Source: CAD feature listing. Evaluate the final solid. Frame: model axes, mm. A direction names the side the tool comes from. Give positions to 0.01 mm unless a question says otherwise; leave off trailing zeros. Loops run counter-clockwise (first coordinate to the right, second up) from the corner with the lowest first, then second, coordinate; pieces in that order, holes last. Notation, with made-up numbers: M 52,-9 L 68,-9 A18 cw 68,21 Z; hole C -20,57 d11. An arc over 180 degrees is marked long. Put each result on its own line as item: value. Start each with the question number.
```python
from build123d import *

# Parameters (mm, degrees)
POSICIONAMENTOS_R               = 6.8994
BASE_DEPTH                      = 3
BASE_DENTE_DEPTH                = 3
RAIO_DENTE_R                    = 0.778916794
PADR_OCIRCULAR1_COUNT           = 10
RAIO_DENTE_OF_PADR_OCIRCULAR1_R = 0.778916794
RESSALTO_EXTRUS_O3_DEPTH        = 3
FURO_DE_DI_METRO_3_0_3_1_D      = 3
FILETE2_R                       = 5
FILETE3_R                       = 13
FILETE4_R                       = 1


with BuildPart() as part:
    # Posicionamentos → Base (new body)
    with BuildSketch(Plane.XY):
        Circle(POSICIONAMENTOS_R)
    extrude(amount=BASE_DEPTH)

    # Dente → Base Dente (add, through all)
    with BuildSketch(Plane.XY):
        with BuildLine():
            Line((1.480256779, 8.326682401), (1.207591527, 6.792896515))
            ThreePointArc((1.207591527, 6.792896515), (0, 6.8994), (-1.207591527, 6.792896515))
            Line((-1.207591527, 6.792896515), (-1.480256779, 8.326682401))
            ThreePointArc((-1.480256779, 8.326682401), (-1.476621376, 8.612123538), (-1.407910185, 8.889195065))
            ThreePointArc((-1.407910185, 8.889195065), (-1.05050148, 9.903958065), (-0.441648539, 10.79096597))
            ThreePointArc((-0.441648539, 10.79096597), (0, 10.8), (0.441648539, 10.79096597))
            ThreePointArc((0.441648539, 10.79096597), (1.05050148, 9.903958065), (1.407910185, 8.889195065))
            ThreePointArc((1.407910185, 8.889195065), (1.476621376, 8.612123538), (1.480256779, 8.326682401))
        make_face()
    base_dente = extrude(amount=BASE_DENTE_DEPTH)

    # Raio Dente
    raio_dente_edges = [part.edges().sort_by_distance(p)[0] for p in [
        (-1.207591527, 6.792896515, 1.5),
        (1.207591527, 6.792896515, 1.5),
    ]]
    fillet(raio_dente_edges, radius=RAIO_DENTE_R)

    # PadrãoCircular1: Base Dente ×10 about axis, 2 skipped
    padr_ocircular1_axis = Axis((0, 0, 0), (0, 0, -1))
    add([base_dente.rotate(padr_ocircular1_axis, i * 360 / PADR_OCIRCULAR1_COUNT) for i in range(1, PADR_OCIRCULAR1_COUNT) if i not in (7, 8)])

    # Raio Dente of PadrãoCircular1
    raio_dente_of_padr_ocircular1_edges = [part.edges().sort_by_distance(p)[0] for p in [
        (3.015802325, 6.205373212, 1.5),
        (4.969726459, 4.785764232, 1.5),
        (6.087262191, 3.247608255, 1.5),
        (6.833594799, 0.950632674, 1.5),
        (6.833594799, -0.950632674, 1.5),
        (6.087262191, -3.247608255, 1.5),
        (4.969726459, -4.785764232, 1.5),
        (3.015802325, -6.205373212, 1.5),
        (1.207591527, -6.792896515, 1.5),
        (-1.207591527, -6.792896515, 1.5),
        (-3.015802325, -6.205373212, 1.5),
        (-4.969726459, -4.785764232, 1.5),
        (-4.969726459, 4.785764232, 1.5),
        (-3.015802325, 6.205373212, 1.5),
    ]]
    fillet(raio_dente_of_padr_ocircular1_edges, radius=RAIO_DENTE_OF_PADR_OCIRCULAR1_R)

    # Braço → Ressalto-extrusão3 (add, through all)
    with BuildSketch(Plane.XY):
        Polygon((0, 4), (-25, 4), (-38, -9), (-25.102702489, -7.416410988), (-21.686291501, -4), (0, -4), align=None)
    extrude(amount=RESSALTO_EXTRUS_O3_DEPTH)

    # Furo de diâmetro Ø3.0 (3)1 (through all)
    with Locations(Plane.XY.offset(3)):
        with Locations((0, 0)):
            Hole(FURO_DE_DI_METRO_3_0_3_1_D / 2)

    # Filete2
    filete2_edges = [part.edges().sort_by_distance(p)[0] for p in [
        (-21.686291501, -4, 1.5),
    ]]
    fillet(filete2_edges, radius=FILETE2_R)

    # Filete3
    filete3_edges = [part.edges().sort_by_distance(p)[0] for p in [
        (-25, 4, 1.5),
    ]]
    fillet(filete3_edges, radius=FILETE3_R)

    # Filete4
    filete4_edges = [part.edges().sort_by_distance(p)[0] for p in [
        (-25.102702489, -7.416410988, 1.5),
        (-38, -9, 1.5),
    ]]
    fillet(filete4_edges, radius=FILETE4_R)


solid = part.part
```
1. Section C-C, the plane y = 2.5. Output: boundary loops of the cut face in (x, z), plus the area to 3 significant figures.
2. Ray query, line 1 (Y direction, x = 0, z = 1.5); line 2 (X direction, y = 4.75, z = 2.2); line 3 (X direction, y = 8.75, z = 1.25). Return the intervals inside material, ascending.
3. Section B-B, the plane x = -17. Output: boundary loops of the cut face in (y, z).
4. Pull-direction query (X, two-part tool) for faces 5 (the face through (-24.66, 2.98, 1.52)), 6 (the face through (-30.35, -8.06, 1.48)), 7 (the face through (10.27, 3.34, 1.48)); classes: released by +X, released by -X, zero draft, split by the parting line, or undercut.
5. Section A-A, the plane x = 0. Output: boundary loops of the cut face in (y, z).
6. Set-up query: faces 1 (the face through (4.985, -8.637, 1.479)), 2 (the face through (-32, -3, 1)), 3 (the face through (1.408, -7.918, 1.479)), 4 (the face through (4.958, 8.623, 1.479)). Return all of +Z, -Z, +X, -X, +Y, -Y with unobstructed straight access to the full face (end or side cutting, diameter ignored); none if empty.
7. Contact query for flat-ended pins moving along their axis: pin 1 (1.5 mm diameter, centred on x = -13, z = 1, fed in from +Y); pin 2 (6 mm diameter, centred on x = -26, y = 7.5, fed in from -Z). Output: stop coordinate, or through.
Results found:
1. outline: M -25.68,0 L 10.13,0 L 10.13,3 L -25.68,3 Z
1. area: 107 mm²
2. line 1: -10.8 to -1.5, 1.5 to 10.8
2. line 2: -5.26 to 5.26
2. line 3: -6.33 to -5.23, -1.45 to 1.45, 5.23 to 6.33
3. outline: M -4,0 L 4,0 L 4,3 L -4,3 Z
4. face 5: released by -X
4. face 6: undercut
4. face 7: released by +X
5. outline: M -10.8,0 L -1.5,0 L -1.5,3 L -10.8,3 Z; M 1.5,0 L 10.8,0 L 10.8,3 L 1.5,3 Z
6. face 1: +Z, -Z, -Y
6. face 2: +Z, -Z, -X, +Y
6. face 3: +Z, -Z
6. face 4: +Z, -Z, +Y
7. pin 1: y = 4
7. pin 2: through
